from build123d import *

# Parameters (mm, degrees)
SKETCH_R        = 74.5
PAD_DEPTH       = 10
SKETCH001_R     = 6.35
POCKET_DEPTH    = 10.001
SKETCH002_R     = 65
SKETCH002_R_2   = 34.5
POCKET001_DEPTH = 6


with BuildPart() as part:
    # Sketch → Pad (new body)
    with BuildSketch(Plane.XZ):
        Circle(SKETCH_R)
    extrude(amount=PAD_DEPTH)

    # Sketch001 (on Face2 of Pad) → Pocket (cut, through all)
    with BuildSketch(Plane(origin=(0, 0, 0), x_dir=(1, 0, 0), z_dir=(0, 1, 0))):
        Circle(SKETCH001_R)
    extrude(amount=-POCKET_DEPTH, mode=Mode.SUBTRACT)

    # Sketch002 (on Face2 of Pocket) → Pocket001 (cut)
    with BuildSketch(Plane(origin=(0, 0, 0), x_dir=(1, 0, 0), z_dir=(0, 1, 0))):
        Circle(SKETCH002_R)
        Circle(SKETCH002_R_2, mode=Mode.SUBTRACT)
    extrude(amount=-POCKET001_DEPTH, mode=Mode.SUBTRACT)


solid = part.part
Source: CAD feature listing. Evaluate the final solid. Frame: model axes, mm. A direction names the side the tool comes from. Round coordinates to 2 decimals unless told otherwise and drop trailing zeros. Loops run counter-clockwise (first coordinate to the right, second up) from the corner with the lowest first, then second, coordinate; pieces in that order, holes last. Notation, with made-up numbers: (75.5, -0.75) -> (101.5, -0.75) arc R11 cw to (101.5, 11.25) -> close; hole circle Ø5 at (-13.75, -22.5). An arc over 180 degrees is marked (long way). Answer as a JSON object with one key per item and string values. Group by question number.
Q1. Section query C-C (y = -3.75). Output: boundary loops of the cut face in (x, z).
Q2. Access query for faces 1 (the cylindrical face through (62, -2.96, -19.52)), 2 (the cylindrical face through (-1.38, -4.93, 6.2)). Directions: +Z, -Z, +X, -X, +Y, -Y. A direction counts if a zero-diameter tool reaches every point of the face in a straight line with its end or side. Return the directions, or none.
Q3. Section query D-D (z = 19). Output: boundary loops of the cut face in (x, y).
Q4. Ray query, line 1 (Z direction, x = 0, y = -5.75); line 2 (X direction, y = -4, z = -8.5); line 3 (Y direction, x = -36, z = 19). Return the intervals inside material, ascending. Write a range as from..to.
Q5. Section query A-A (x = 0). Output: boundary loops of the cut face in (y, z), plus the area to 3 significant figures.
Q6. Contact query for flat-ended pins moving along their axis: P1, Ø1.5, axis at x = 56.5, y = -6.5, coming from the +Z side; P2, Ø5, axis at x = -52, z = 40, coming from the +Y side; P3, Ø5, axis at x = 3, y = -4, coming from the +Z side. Output: stop coordinate, or through.
Q7. Mould query, pull axis X, two halves, no side actions, for faces 3 (the cylindrical face through (32.907, -2.958, -10.363)), 4 (the flat face through (5, 0, 67)), 5 (the cylindrical face through (71.06, -4.93, 22.38)). Classes: pulls with the +X half, pulls with the -X half, needs draft (parallel to the pull), parting line crosses it, or undercut.
Q8. Section query B-B (z = 0). Output: boundary loops of the cut face in (x, y).
Completed:
{
 "1": {"outline": "circle Ø149 at (0, 0); circle Ø69 at (0, 0); hole circle Ø130 at (0, 0); hole circle Ø12.7 at (0, 0)"},
 "2": {"face 1": "+Y", "face 2": "+Y, -Y"},
 "3": {"outline": "(-72.04, -10) -> (72.04, -10) -> (72.04, 0) -> (62.16, 0) -> (62.16, -6) -> (28.8, -6) -> (28.8, 0) -> (-28.8, 0) -> (-28.8, -6) -> (-62.16, -6) -> (-62.16, 0) -> (-72.04, 0) -> close"},
 "4": {"line 1": "-74.5..-65, -34.5..-6.35, 6.35..34.5, 65..74.5", "line 2": "-74.01..-64.44, -33.44..33.44, 64.44..74.01", "line 3": "-10..-6"},
 "5": {"outline": "(-10, -74.5) -> (0, -74.5) -> (0, -65) -> (-6, -65) -> (-6, -34.5) -> (0, -34.5) -> (0, -6.35) -> (-10, -6.35) -> close; (-10, 6.35) -> (0, 6.35) -> (0, 34.5) -> (-6, 34.5) -> (-6, 65) -> (0, 65) -> (0, 74.5) -> (-10, 74.5) -> close", "area": "997 mm²"},
 "6": {"P1": "z = 49.42", "P2": "y = 0", "P3": "z = 74.5"},
 "7": {"face 3": "undercut", "face 4": "needs draft", "face 5": "parting line crosses it"},
 "8": {"outline": "(-74.5, -10) -> (-6.35, -10) -> (-6.35, 0) -> (-34.5, 0) -> (-34.5, -6) -> (-65, -6) -> (-65, 0) -> (-74.5, 0) -> close; (6.35, -10) -> (74.5, -10) -> (74.5, 0) -> (65, 0) -> (65, -6) -> (34.5, -6) -> (34.5, 0) -> (6.35, 0) -> close"}
}
